Part model, mm, in its own coordinate system. Face numbers are marked on the shaded views. Give positions to 0.01 mm unless a question says otherwise; leave off trailing zeros. Loops run counter-clockwise (first coordinate to the right, second up) from the corner with the lowest first, then second, coordinate; pieces in that order, holes last. Notation, with made-up numbers: (88.5, -19) -> (147.5, -19) arc R16 ccw to (147.5, -8) -> close; hole circle Ø6 at (9.5, 48.5). An arc over 180 degrees is marked (long way). Write item = value, one per line.
Autodesk Inventor part; units mm, degrees
ref_plane "YZ Plane" through (0, 0, 0) normal (1, 0, 0) x (0, 1, 0)
ref_plane "XZ Plane" through (0, 0, 0) normal (0, 1, 0) x (-1, 0, 0)
ref_plane "XY Plane" through (0, 0, 0) normal (0, 0, 1) x (1, 0, 0)
ref_plane "Work Plane1" through (-0.0001, 0, -396.2798) normal (0, 0, 1) x (1, 0, 0)
sketch "Sketch1" plane through (-0.0001, 0, -396.2798) normal (0, 0, 1) x (1, 0, 0)
  circle A0 centre (29.9617, 10.0469) radius 2.1
  circle A1 centre (29.9617, -9.9531) radius 2.1
  circle A2 centre (-30.0383, -9.9531) radius 2.1
  circle A3 centre (-30.0383, 10.0469) radius 2.1
  circle A4 centre (-10.0383, -9.9531) radius 2.1
  circle A5 centre (9.9617, -9.9531) radius 2.1
  line L0 (39.9617, 19.5469) -> (39.9617, 14.8783)
  line L1 (39.9617, -14.7846) -> (39.9617, -19.4531)
  line L2 (39.4617, -19.9531) -> (34.7932, -19.9531)
  line L3 (20.4617, 20.0469) -> (25.0617, 20.0469)
  line L4 (-34.8697, -19.9531) -> (-39.5383, -19.9531)
  line L5 (-40.0383, 14.8783) -> (-40.0383, 19.5469)
  line L6 (-39.5383, 20.0469) -> (-34.9383, 20.0469)
  line L7 (-40.0383, -19.4531) -> (-40.0383, -14.7846)
  line L8 (39.9617, 20.0469) -> (39.9617, -19.9532) construction
  line L9 (39.9617, -19.9532) -> (-40.0383, -19.9531) construction
  line L10 (-40.0383, -19.9531) -> (-40.0383, 20.0469) construction
  line L11 (-20.0383, 19.5469) -> (-20.0383, 14.8783)
  line L12 (19.9617, 0.0469) -> (19.9617, 5.2154)
  line L13 (-20.0383, 0.0469) -> (-14.9383, 0.0469)
  line L14 (39.9617, 20.0469) -> (19.9617, 20.0469) construction
  line L15 (19.9617, 20.0469) -> (19.9617, 0.0469) construction
  line L16 (-20.0383, 0.0469) -> (19.9617, 0.0469) construction
  line L17 (-40.0383, 20.0469) -> (-20.0383, 20.0469) construction
  line L18 (-20.0383, 20.0469) -> (-20.0383, 0.0469) construction
  line L19 (45.6493, 27.0762) -> (45.6493, -26.9238)
  line L20 (-64.252, 0) -> (79.446, 0) construction
  line L21 (18.0586, 45.1257) -> (28.1307, -1.0304) construction
  line L22 (28.1307, -1.0304) -> (-18.0254, -11.1025) construction
  circle A6 centre (28.1307, -1.0304) radius 2.55
  circle A7 centre (-18.0452, -9.0596) radius 2.55
  circle A8 centre (18.0586, 45.1257) radius 2.55
  circle A9 centre (-18.0452, -9.0596) radius 3.5 construction
  circle A10 centre (18.0586, 45.1257) radius 3.5 construction
  circle A11 centre (28.1307, -1.0304) radius 3.5 construction
  line L23 (48.593, 17.0469) -> (-85.0986, 17.0469) construction
  line L24 (-0.0383, 40.3857) -> (-0.0383, -33.3677) construction
  circle A12 centre (-0.0383, 17.0469) radius 11.05
  line L25 (31.6013, 44.4325) -> (22.7125, 55.4148)
  line L26 (22.7125, 55.4148) -> (5.0035, 55.4148)
  line L27 (5.0035, 55.4148) -> (-5.8027, 44.4325)
  line L28 (-64.3507, 44.498) -> (-5.8027, 44.4325)
  line L29 (-64.3507, 44.498) -> (-66.5209, 44.5005)
  line L30 (-55.0383, 44.4876) -> (-55.0383, -55.6033) construction
  line L31 (45.6493, -26.9238) -> (-85.0986, -26.7776)
  line L32 (45.6493, -26.9238) -> (185.0342, -26.9238) construction
  line L33 (40.0498, -55.6502) -> (39.9617, -55.6502)
  line L34 (-83.2302, 44.5192) -> (-66.5209, 44.5005)
  line L35 (-85.0986, -26.7776) -> (-85.0986, 44.5192)
  line L36 (-85.0986, 44.5192) -> (-83.2302, 44.5192)
  line L37 (-5.8027, 44.4325) -> (31.6013, 44.4325) construction
  line L38 (31.6013, 44.4325) -> (45.6493, 44.4325)
  line L39 (45.6493, 44.4325) -> (45.6493, 27.0762)
  point P0 (0, 0)
  point P1 (0, 17)
  point P2 (22.7617, 20.0469)
  point P3 (19.9617, 2.6311)
  point P4 (-40.0383, -17.1189)
  point P5 (-55.0383, -5.5579)
  point P6 (-75.0383, 17.0469)
  point P7 (-55.0383, 17.0469)
  dimension "d2" = 110
  dimension "d3" = 5.1
  dimension "d4" = 5.1
  dimension "d5" = 5.1
  dimension "d7" = 7
  dimension "d8" = 7
  dimension "d9" = 7
  dimension "d10" = 3
  dimension "d11" = 20
  dimension "d12" = 22.1
  dimension "d30" = 15
  dimension "d33" = 54
  dimension "d36" = 20
  dimension "d37" = 15
extrude "Extrusion1" add sketch "Sketch1" along normal blind 6 contours A0 | A1 | A2 | A3 | A4 | A5 | L19 L31 L35 L36 L34 L29 L28 L27 L26 L25 L38 L39 | A6 | A7 | A8
sketch "Sketch2" plane through (-0.0001, 0, -396.2798) normal (0, 0, -1) x (-1, 0, 0)
  point P0 (0, 0)
  point P1 (-29.9617, -9.9531)
  point P2 (-10.0691, -10.0439)
  point P3 (9.9252, -10.1028)
  point P4 (18.1169, -8.9461)
  point P5 (29.8554, -9.9987)
  point P6 (30.0649, 10.1011)
  point P7 (-30.1907, 10.308)
  point P8 (-18.3441, 44.9518)
  point P9 (55.0383, 17.0469)
  point P10 (75.0383, 17.0469)
hole "Hole1" at (29.9617, -9.9531, -396.2798) at (10.0691, -10.0439, -396.2798) at (-18.1169, -8.9461, -396.2798) at (-29.8554, -9.9987, -396.2798) at (-30.065, 10.1011, -396.2798) at (30.1907, 10.308, -396.2798) at (18.344, 44.9518, -396.2798) at (-75.0383, 17.0468, -396.2798) at (-55.0383, 17.0468, -396.2798) direction (0, 0, 1) diameter 5.1 end through all
properties part number "X axis motor mount_3DPrint"
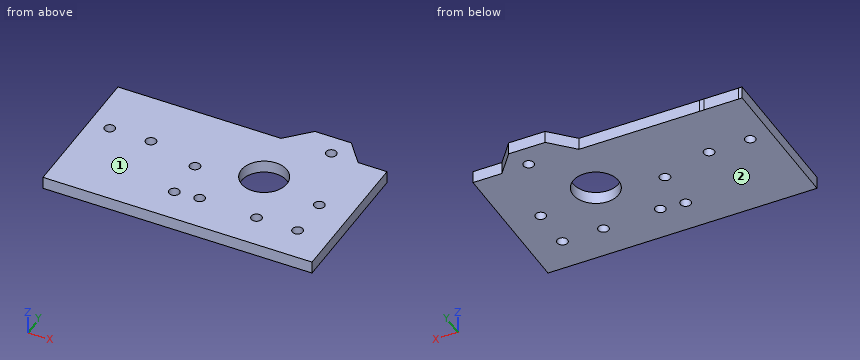
1) Slice it at B-B, the plane y = 10.5. List the corners of the cut face in (x, z), and give its area (3 significant figures).
Resolved:
outline = (-85.1, -396.28) -> (-32.58, -396.28) -> (-32.58, -390.28) -> (-85.1, -390.28) -> close; (-27.55, -396.28) -> (-8.94, -396.28) -> (-8.94, -390.28) -> (-27.55, -390.28) -> close; (8.86, -396.28) -> (27.65, -396.28) -> (27.65, -390.28) -> (8.86, -390.28) -> close; (32.73, -396.28) -> (45.65, -396.28) -> (45.65, -390.28) -> (32.73, -390.28) -> close
area = 617 mm²
2) Drill centre lines: line 1 along Y through (x, z) = (30, -395.1); line 2 along X through (y, z) = (18, -392.1); line 3 along X through (y, z) = (19, -390.65). Where is each one in solid material? Low to high. Write a range as [from, to].
Resolved:
line_1 = [-26.91, -12.5], [-7.4, 7.77], [12.85, 46.41]
line_2 = [-85.1, -77.4], [-72.67, -57.4], [-52.67, -11.05], [10.97, 45.65]
line_3 = [-85.1, -76.68], [-73.4, -56.68], [-53.4, -10.91], [10.84, 45.65]
3) Pull direction Z, two halves, no side cores. Call the marked faces 1 and 2: pulls with the +Z half, pulls with the -Z half, needs draft (parallel to the pull), parting line crosses it, or undercut.
Resolved:
face_1 = pulls with the +Z half
face_2 = pulls with the -Z half
4) Drop flat-ended pins along their axis: P1, Ø6.5, axis at x = -55.04, y = 17.05, coming from the +Z side; P2, Ø4, axis at x = -75.04, y = 17.05, coming from the -Z side; P3, Ø0.6, axis at x = -84.5, z = -394, coming from the +Y side. Give the stop position or say it passes through.
Resolved:
P1 = -390.28
P2 = through
P3 = 44.52
5) Slice it at D-D, the plane x = -39.5. List the corners of the cut face in (y, z), and give its area (3 significant figures).
Resolved:
outline = (-26.83, -396.28) -> (44.47, -396.28) -> (44.47, -390.28) -> (-26.83, -390.28) -> close
area = 428 mm²
6) Slice it at C-C, the plane x = 34.5. List the corners of the cut face in (y, z), and give its area (3 significant figures).
Resolved:
outline = (-26.91, -396.28) -> (44.43, -396.28) -> (44.43, -390.28) -> (-26.91, -390.28) -> close
area = 428 mm²
7) Slice it at A-A, the plane z = -391.75. Count the separate pieces of the cut face and the enclosed holes in it, and give its area (3 significant figures).
Resolved:
separate_pieces = 1
enclosed_holes = 10
area = 9,060 mm²
